```python
from build123d import *

# Parameters (mm, degrees)
EXTRUDE_1_DEPTH     = 26
EXTRUDE_START       = 2
EXTRUDE_2_DEPTH     = 2
EXTRUDE_3_DEPTH     = 2
SKETCH_7_W          = 6.5
SKETCH_7_H          = 34
SKETCH_7_R          = 1.6
SKETCH_7_R_2        = 1.25
EXTRUDE_4_DEPTH     = 6
FILLET_1_R          = 2
EXTRUDE_5_REACH     = 58.145
SKETCH_9_R          = 3
SKETCH_9_R_2        = 1.35
SKETCH_10_R         = 2.75
CUT_EXTRUDE_1_DEPTH = 2.5
CUT_EXTRUDE_4_DEPTH = 26


with BuildPart() as part:
    # 草图2 → 凸台-拉伸1 (new, symmetric)
    with BuildSketch(Plane(origin=(0, 0, 0), x_dir=(0, 0, -1), z_dir=(1, 0, 0))):
        with BuildLine():
            Line((0, 34.014702703), (0, 39))
            Line((0, 39), (2.5, 39))
            Line((2.5, 39), (2.5, 35))
            ThreePointArc((2.5, 35), (15.52803004, 0), (2.5, -35))
            Line((2.5, -35), (2.5, -39))
            Line((2.5, -39), (0, -39))
            Line((0, -39), (0, -34.014702703))
            ThreePointArc((0, -34.014702703), (13, 0), (0, 34.014702703))
        make_face()
    extrude(amount=EXTRUDE_1_DEPTH, both=True)

    # 草图3 → 凸台-拉伸2 (add)
    with BuildSketch(Plane(origin=(26, 0, 0), x_dir=(0, 0, -1), z_dir=(1, 0, 0)).offset(EXTRUDE_START)):
        with BuildLine():
            Line((0, 39), (0, -39))
            Line((0, -39), (2.5, -39))
            Line((2.5, -39), (2.5, -35))
            ThreePointArc((2.5, -35), (15.52803004, 0), (2.5, 35))
            Line((2.5, 35), (2.5, 39))
            Line((2.5, 39), (0, 39))
        make_face()
    extrude(amount=-EXTRUDE_2_DEPTH)

    # 草图4 → 凸台-拉伸3 (add)
    with BuildSketch(Plane.ZY.offset(26)):
        with BuildLine():
            Line((-2.5, 35), (-2.5, 39))
            Line((-2.5, 39), (0, 39))
            Line((0, 39), (0, -39))
            Line((0, -39), (-2.5, -39))
            Line((-2.5, -39), (-2.5, -35))
            ThreePointArc((-2.5, -35), (-15.52803004, 0), (-2.5, 35))
        make_face()
    extrude(amount=EXTRUDE_3_DEPTH)

    # 草图7 → 凸台-拉伸4 (add)
    # profile 1 of 2: a face of its own
    with BuildSketch(Plane.XY):
        with Locations((31.25, 0)):
            Rectangle(SKETCH_7_W, SKETCH_7_H)
        with Locations((31, 0)):
            Circle(SKETCH_7_R, mode=Mode.SUBTRACT)
        with Locations((31, 13)):
            Circle(SKETCH_7_R_2, mode=Mode.SUBTRACT)
        with Locations(Location((31, -13, 0), (0, 0, 180))):
            Circle(SKETCH_7_R_2, mode=Mode.SUBTRACT)
    # profile 2 of 2: a face of its own
    with BuildSketch(Plane.XY):
        with Locations((-31.25, 0)):
            Rectangle(SKETCH_7_W, SKETCH_7_H)
        with Locations((-31, -13)):
            Circle(SKETCH_7_R_2, mode=Mode.SUBTRACT)
        with Locations(Location((-31, 0, 0), (0, 0, 180))):
            Circle(SKETCH_7_R, mode=Mode.SUBTRACT)
        with Locations(Location((-31, 13, 0), (0, 0, 180))):
            Circle(SKETCH_7_R_2, mode=Mode.SUBTRACT)
    extrude(amount=-EXTRUDE_4_DEPTH)

    # 圆角1
    fillet_1_edges = [part.edges().sort_by_distance(p)[0] for p in [
        (28, -17, -3),
        (28, 17, -3),
        (34.5, 17, -3),
        (34.5, -17, -3),
        (-34.5, -17, -3),
        (-34.5, 17, -3),
        (-28, 17, -3),
        (-28, -17, -3),
    ]]
    fillet(fillet_1_edges, radius=FILLET_1_R)

    # 凸台-拉伸5: up to this face of the body (flat: up to its plane)
    extrude_5_end = Plane(part.part.faces().sort_by_distance((0, 37, -2.5))[0])
    # 草图9 → 凸台-拉伸5 (add, up to the picked face)
    with BuildSketch(Plane.XY.offset(-21), mode=Mode.PRIVATE) as extrude_5_sk1:
        with Locations(Location((-24.765, 32.705, 0), (0, 0, 130.093007985))):
            Circle(SKETCH_9_R)
        with Locations(Location((-24.765, 32.705, 0), (0, 0, 180))):
            Circle(SKETCH_9_R_2, mode=Mode.SUBTRACT)
    extrude_5_tool1 = split(extrude(extrude_5_sk1.sketch, amount=EXTRUDE_5_REACH, mode=Mode.PRIVATE), bisect_by=extrude_5_end, keep=Keep.BOTH, mode=Mode.PRIVATE)
    # 草图9 → 凸台-拉伸5 (add, up to the picked face)
    with BuildSketch(Plane.XY.offset(-21), mode=Mode.PRIVATE) as extrude_5_sk2:
        with Locations(Location((24.765, 32.705, 0), (0, 0, 180))):
            Circle(SKETCH_9_R)
        with Locations(Location((24.765, 32.705, 0), (0, 0, 180))):
            Circle(SKETCH_9_R_2, mode=Mode.SUBTRACT)
    extrude_5_tool2 = split(extrude(extrude_5_sk2.sketch, amount=EXTRUDE_5_REACH, mode=Mode.PRIVATE), bisect_by=extrude_5_end, keep=Keep.BOTH, mode=Mode.PRIVATE)
    # 草图9 → 凸台-拉伸5 (add, up to the picked face)
    with BuildSketch(Plane.XY.offset(-21), mode=Mode.PRIVATE) as extrude_5_sk3:
        with Locations(Location((24.765, -32.705, 0), (0, 0, 229.906992015))):
            Circle(SKETCH_9_R)
        with Locations(Location((24.765, -32.705, 0), (0, 0, 180))):
            Circle(SKETCH_9_R_2, mode=Mode.SUBTRACT)
    extrude_5_tool3 = split(extrude(extrude_5_sk3.sketch, amount=EXTRUDE_5_REACH, mode=Mode.PRIVATE), bisect_by=extrude_5_end, keep=Keep.BOTH, mode=Mode.PRIVATE)
    # 草图9 → 凸台-拉伸5 (add, up to the picked face)
    with BuildSketch(Plane.XY.offset(-21), mode=Mode.PRIVATE) as extrude_5_sk4:
        with Locations(Location((-24.765, -32.705, 0), (0, 0, 180))):
            Circle(SKETCH_9_R)
        with Locations(Location((-24.765, -32.705, 0), (0, 0, 180))):
            Circle(SKETCH_9_R_2, mode=Mode.SUBTRACT)
    extrude_5_tool4 = split(extrude(extrude_5_sk4.sketch, amount=EXTRUDE_5_REACH, mode=Mode.PRIVATE), bisect_by=extrude_5_end, keep=Keep.BOTH, mode=Mode.PRIVATE)
    add(extrude_5_tool1.solids().sort_by(Axis((-22.887557, 30.474912, -21), (0, 0, 1)))[0])
    add(extrude_5_tool2.solids().sort_by(Axis((27.680147, 32.705, -21), (0, 0, 1)))[0])
    add(extrude_5_tool3.solids().sort_by(Axis((26.642443, -30.474912, -21), (0, 0, 1)))[0])
    add(extrude_5_tool4.solids().sort_by(Axis((-21.849853, -32.705, -21), (0, 0, 1)))[0])

    # 草图10 → 切除-拉伸1 (cut)
    with BuildSketch(Plane.XY):
        with Locations((-31, 0)):
            Circle(SKETCH_10_R)
        with Locations((31, 0)):
            Circle(SKETCH_10_R)
    extrude(amount=-CUT_EXTRUDE_1_DEPTH, mode=Mode.SUBTRACT)

    # 草图12 → 切除-拉伸4 (cut, symmetric)
    with BuildSketch(Plane(origin=(0, 0, 0), x_dir=(0, 0, -1), z_dir=(1, 0, 0))):
        with BuildLine():
            Line((0, 34.014702703), (0, -34.014702703))
            ThreePointArc((0, -34.014702703), (13, 0), (0, 34.014702703))
        make_face()
    extrude(amount=CUT_EXTRUDE_4_DEPTH, both=True, mode=Mode.SUBTRACT)


solid = part.part
```
Work out the finished part from the listing and answer in its coordinate system (mm). A direction names the side the tool comes from. Coordinates: 2 decimals unless noted, no trailing zeros. Loops run counter-clockwise (first coordinate to the right, second up) from the corner with the lowest first, then second, coordinate; pieces in that order, holes last.
1) Section C-C (x = -31) is taken. Give the vertices of the cut face in (y, z), plus the area to 3 significant figures.
Results:
outline: (-17, -6) - (-14.25, -6) - (-14.25, 0) - (-17, 0) - close; (-11.75, -6) - (-1.6, -6) - (-1.6, -2.5) - (-2.75, -2.5) - (-2.75, 0) - (-11.75, 0) - close; (1.6, -6) - (11.75, -6) - (11.75, 0) - (2.75, 0) - (2.75, -2.5) - (1.6, -2.5) - close; (14.25, -6) - (17, -6) - (17, 0) - (14.25, 0) - close
area: 149 mm2
2) Section A-A (y = 0) is taken. Give the vertices of the cut face in (x, z), plus the area to 3 significant figures.
Results:
outline: (-34.5, -6) - (-32.6, -6) - (-32.6, -2.5) - (-33.75, -2.5) - (-33.75, 0) - (-34.5, 0) - close; (-29.4, -6) - (-28, -6) - (-28, -15.53) - (28, -15.53) - (28, -6) - (29.4, -6) - (29.4, -2.5) - (28.25, -2.5) - (28.25, 0) - (26, 0) - (26, -13) - (-26, -13) - (-26, 0) - (-28.25, 0) - (-28.25, -2.5) - (-29.4, -2.5) - close; (32.6, -6) - (34.5, -6) - (34.5, 0) - (33.75, 0) - (33.75, -2.5) - (32.6, -2.5) - close
area: 222 mm2
3) Section B-B (z = -17.5) is taken. Give the vertices of the cut face in (x, y) (3 decimals), plus the area to 3 significant figures.
Results:
outline: circle Ø6 at (-24.765, -32.705); circle Ø6 at (-24.765, 32.705); circle Ø6 at (24.765, -32.705); circle Ø6 at (24.765, 32.705); hole circle Ø2.7 at (-24.765, -32.705); hole circle Ø2.7 at (-24.765, 32.705); hole circle Ø2.7 at (24.765, -32.705); hole circle Ø2.7 at (24.765, 32.705)
area: 90.2 mm2
4) For faces 4 (the flat face through (-29, 0, -2.5)), 5 (the flat face through (31, -17, -3)), 6 (the cylindrical face through (24.941, -34.044, -12.273)), determine the directions among +Z, -Z, +X, -X, +Y, -Y from which every point of the face is accessible in a straight line to the end or side of a thin tool.
Results:
face 4: +Z
face 5: +Z, -Z, +X, -Y
face 6: -Z
5) For a pull along Y with two mould halves and no side action, classify faces 1 (the cylindrical face through (24.79, 32.7, -4.38)), 2 (the cylindrical face through (-33.9, -16.43, -3.04)), 3 (the flat face through (-28, 0, 0)) as +Y half, -Y half, draft (parallel to the pull), parting line (faces both ways), or undercut.
Results:
face 1: undercut
face 2: -Y half
face 3: draft
6) Consider probe 1 along Y at (x, z) = (31, -3.4); probe 2 along Y at (x, z) = (-31, -2.45); probe 3 along X at (y, z) = (19, -5.5). Determine where each line is inside the solid, lowest interval first.
Results:
probe 1: y = -17 to -14.25, -11.75 to -1.6, 1.6 to 11.75, 14.25 to 17
probe 2: y = -17 to -14.25, -11.75 to -2.75, 2.75 to 11.75, 14.25 to 17
probe 3: x = -28 to -26, 26 to 28
7) Section D-D (x = 8.5) is taken. Give the vertices of the cut face in (y, z), plus the area to 3 significant figures.
Results:
outline: (-39, -2.5) - (-35, -2.5) arc R53.53 ccw to (35, -2.5) - (39, -2.5) - (39, 0) - (34.01, 0) arc R51 cw to (-34.01, 0) - (-39, 0) - close
area: 213 mm2
8) Flat-ended cylindrical pins translate along their axes: pin 1 (3 mm diameter, centred on x = 31.5, z = -2, fed in from +Y); pin 2 (5 mm diameter, centred on x = 17, y = -15, fed in from +Z); pin 3 (1.5 mm diameter, centred on x = 18, y = 17, fed in from -Z); pin 4 (1.6 mm diameter, centred on x = -31.5, y = 0.5, fed in from +Z). Find the tip coordinate at first contact, or state that the pin passes through.
Results:
pin 1: stops at y = 17
pin 2: stops at z = -9.9
pin 3: stops at z = -13
pin 4: passes through
